Geometry check sheet. Reference: the model listing, model coordinates, mm. A direction names the side the tool comes from. Give positions to 0.01 mm unless a question says otherwise; leave off trailing zeros. Loops run counter-clockwise (first coordinate to the right, second up) from the corner with the lowest first, then second, coordinate; pieces in that order, holes last. Notation, with made-up numbers: (87, 79.25) -> (140, 79.25) arc R29 cw to (140, 101.25) -> close; hole circle Ø8 at (30, -13.75). An arc over 180 degrees is marked (long way). One line per item, written item: value. Start each with the question number.
(1) Sectioned sample at D-D, the plane x = 5.5. Record the cut outline in (y, z).
(2) Tool access check on faces 4 (the face through (6.384, 1.232, -6.232)), 5 (the face through (1.5, 1.2, -2.6)). Record the directions out of +Z, -Z, +X, -X, +Y, -Y that give a thin tool (end or side, any length) a straight path to the whole face; none if there is none.
(3) Sectioned sample at B-B, the plane z = -9. Record the cut outline in (x, y).
(4) Sectioned sample at C-C, the plane y = 0.85. State how many separate pieces and enclosed holes the cut face has, then the cut area to 3 significant figures.
(5) Sectioned sample at A-A, the plane x = 10. Record the cut outline in (y, z).
(6) Scan lines: line 1 along Z through (x, y) = (10, 1.85); line 2 along Z through (x, y) = (4.75, 1.95); line 3 along Z through (x, y) = (2.5, 0.35). Record each from-to range of solid material in increasing order. Write a range as from..to.
(7) Draft check along X on faces 1 (the face through (9, 1, 0)), 2 (the face through (8.1, 1.23, -7.26)), 3 (the face through (0, 1, -8)). Enter one of: pulls with the +X half, pulls with the -X half, needs draft (parallel to the pull), parting line crosses it, or undercut.
from build123d import *

# Parameters (mm, degrees)
SKETCH1_W             = 14.482050808
SKETCH1_H             = 16.660254038
BOSS_EXTRUDE1_DEPTH   = 2.5
CHAMFER1_SIZE         = 3
CHAMFER1_SIZE2        = 5.196152423
CHAMFER1_PART_2_SIZE  = 3
CHAMFER1_PART_2_SIZE2 = 5.196152423


with BuildPart() as part:
    # Sketch1 → Boss-Extrude1 (new body)
    with BuildSketch(Plane(origin=(0, 0, 0), x_dir=(1, 0, 0), z_dir=(0, 1, 0))):
        with Locations((7.241025404, 8.330127019)):
            Rectangle(SKETCH1_W, SKETCH1_H)
        Polygon((7.482050808, 14.660254038), (12.482050808, 14.660254038), (11.232050808, 12.495190528), (8.732050808, 12.495190528), align=None, mode=Mode.SUBTRACT)
        Polygon((7, 11.495190528), (5.75, 13.660254038), (3.25, 13.660254038), (2, 11.495190528), (3.25, 9.330127019), (5.75, 9.330127019), align=None, mode=Mode.SUBTRACT)
        Polygon((7, 5.165063509), (5.75, 7.330127019), (3.25, 7.330127019), (2, 5.165063509), (3.25, 3), (5.75, 3), align=None, mode=Mode.SUBTRACT)
        Polygon((12.482050808, 8.330127019), (11.232050808, 10.495190528), (8.732050808, 10.495190528), (7.482050808, 8.330127019), (8.732050808, 6.165063509), (11.232050808, 6.165063509), align=None, mode=Mode.SUBTRACT)
        Polygon((7.482050808, 2), (12.482050808, 2), (11.232050808, 4.165063509), (8.732050808, 4.165063509), align=None, mode=Mode.SUBTRACT)
    extrude(amount=BOSS_EXTRUDE1_DEPTH)

    # Chamfer1
    chamfer1_edges = [part.edges().sort_by_distance(p)[0] for p in [
        (0, 1.25, -16.660254038),
    ]]
    chamfer1_side = [part.faces().sort_by_distance(p)[0] for p in [
        (7.241025404, 1.25, -16.660254038),
    ]]
    chamfer(chamfer1_edges, length=CHAMFER1_SIZE, length2=CHAMFER1_SIZE2, reference=chamfer1_side[0])

    # Chamfer1 part 2
    chamfer1_part_2_edges = [part.edges().sort_by_distance(p)[0] for p in [
        (0, 1.25, 0),
    ]]
    chamfer1_part_2_side = [part.faces().sort_by_distance(p)[0] for p in [
        (7.241025404, 1.25, 0),
    ]]
    chamfer(chamfer1_part_2_edges, length=CHAMFER1_PART_2_SIZE, length2=CHAMFER1_PART_2_SIZE2, reference=chamfer1_part_2_side[0])


solid = part.part
Calculated:
1. outline: (0, -16.66) -> (2.5, -16.66) -> (2.5, -13.66) -> (0, -13.66) -> close; (0, -9.33) -> (2.5, -9.33) -> (2.5, -7.33) -> (0, -7.33) -> close; (0, -3) -> (2.5, -3) -> (2.5, 0) -> (0, 0) -> close
2. face 4: +Y, -Y
2. face 5: +Z, -X, +Y, -Y
3. outline: (0, 0) -> (7.87, 0) -> (7.87, 2.5) -> (0, 2.5) -> close; (12.1, 0) -> (14.48, 0) -> (14.48, 2.5) -> (12.1, 2.5) -> close
4. separate pieces: 1
4. enclosed holes: 5
4. area: 161 mm2
5. outline: (0, -16.66) -> (2.5, -16.66) -> (2.5, -14.66) -> (0, -14.66) -> close; (0, -12.5) -> (2.5, -12.5) -> (2.5, -10.5) -> (0, -10.5) -> close; (0, -6.17) -> (2.5, -6.17) -> (2.5, -4.17) -> (0, -4.17) -> close; (0, -2) -> (2.5, -2) -> (2.5, 0) -> (0, 0) -> close
6. line 1: z = -16.66..-14.66, -12.5..-10.5, -6.17..-4.17, -2..0
6. line 2: z = -16.66..-13.66, -9.33..-7.33, -3..0
6. line 3: z = -15.79..-12.36, -10.63..-6.03, -4.3..-0.87
7. face 1: needs draft
7. face 2: undercut
7. face 3: pulls with the -X half
